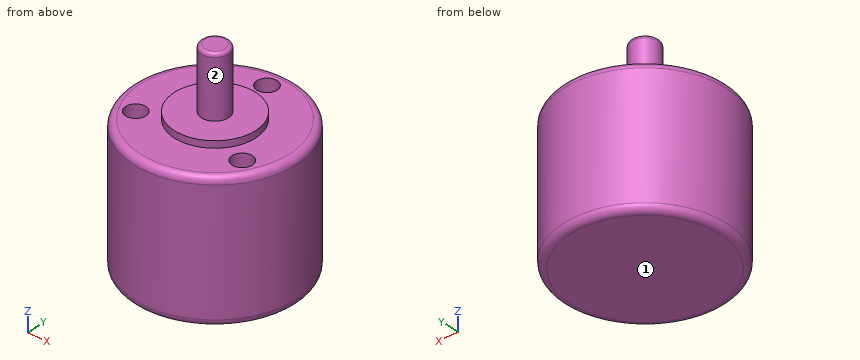
```python
from build123d import *

# Parameters (mm, degrees)
ESQUISSE1_R             = 12
EXTRUSION1_DEPTH        = 20
ESQUISSE2_R             = 2
EXTRUSION2_DEPTH        = 10
CONG_1_R                = 1
CONG_2_R                = 1
CONG_3_R                = 0.5
ESQUISSE4_R             = 6
EXTRUSION3_DEPTH        = 1
ESQUISSE5_R             = 1.5
ENL_V_MAT_EXTRU_1_DEPTH = 5


with BuildPart() as part:
    # Esquisse1 → Extrusion1 (new body)
    with BuildSketch(Plane.XY):
        Circle(ESQUISSE1_R)
    extrude(amount=-EXTRUSION1_DEPTH)

    # Esquisse2 → Extrusion2 (add)
    with BuildSketch(Plane.XY):
        Circle(ESQUISSE2_R)
    extrude(amount=EXTRUSION2_DEPTH)

    # Congé1
    cong_1_edges = [part.edges().sort_by_distance(p)[0] for p in [
        (-12, 0, 0),
    ]]
    fillet(cong_1_edges, radius=CONG_1_R)

    # Congé2
    cong_2_edges = [part.edges().sort_by_distance(p)[0] for p in [
        (-12, 0, -20),
    ]]
    fillet(cong_2_edges, radius=CONG_2_R)

    # Congé3
    cong_3_edges = [part.edges().sort_by_distance(p)[0] for p in [
        (-2, 0, 10),
    ]]
    fillet(cong_3_edges, radius=CONG_3_R)

    # Esquisse4 → Extrusion3 (add)
    with BuildSketch(Plane.XY):
        Circle(ESQUISSE4_R)
    extrude(amount=EXTRUSION3_DEPTH)

    # Esquisse5 → Enlèv. mat.-Extru.1 (cut)
    with BuildSketch(Plane.XY):
        with Locations((0, 9)):
            Circle(ESQUISSE5_R)
        with Locations((-7.794228634, -4.5)):
            Circle(ESQUISSE5_R)
        with Locations((7.794228634, -4.5)):
            Circle(ESQUISSE5_R)
    extrude(amount=-ENL_V_MAT_EXTRU_1_DEPTH, mode=Mode.SUBTRACT)


solid = part.part
```
Check sheet for the modelled part. Datum: model origin and axes. Units: mm. Face numbers are marked on the shaded views. A direction names the side the tool comes from. Round coordinates to 2 decimals unless told otherwise and drop trailing zeros. Loops run counter-clockwise (first coordinate to the right, second up) from the corner with the lowest first, then second, coordinate; pieces in that order, holes last. Notation, with made-up numbers: (-20, 56) - (23, 56) arc R13 cw to (23, 77) - close; hole circle Ø5 at (15.5, 79.5). An arc over 180 degrees is marked (long way). Answer as a JSON object with one key per item and string values. Group by question number.
Q1. Sectioned sample at C-C, the plane z = 8. Enter the section's corners in (x, y), plus the area to 3 significant figures.
Q2. Gauge pin test, flat ends, axial feed: P1, Ø8, axis at y = 9, z = -11, coming from the -X side; P2, Ø12, axis at x = -8.5, y = -0.5, coming from the +Z side; P3, Ø1, axis at x = -6.5, y = 5, coming from the +Z side. Record the tip position at first contact, or that the pin passes through.
Q3. Scan lines: line 1 along Y through (x, z) = (0, -3.2); line 2 along Y through (x, z) = (0, -18.75); line 3 along Z through (x, y) = (-3.25, -1.5). Record each from-to range of solid material in increasing order. Write a range as [from, to].
Q4. Sectioned sample at B-B, the plane y = 0. Enter the section's corners in (x, z).
Q5. Set-up check for the marked faces 1 and 2: record each of +Z, -Z, +X, -X, +Y, -Y from which the full face is reachable in a straight line by a thin tool's end or side.
Q6. Sectioned sample at A-A, the plane z = -2.75. Enter the section's corners in (x, y), plus the area to 3 significant figures.
Solution:
{
 "1": {"outline": "circle Ø4 at (0, 0)", "area": "12.6 mm²"},
 "2": {"P1": "stops at x = -10.91", "P2": "stops at z = 1", "P3": "stops at z = 0"},
 "3": {"line 1": "y = [-12, 7.5], [10.5, 12]", "line 2": "y = [-12, 12]", "line 3": "z = [-20, 1]"},
 "4": {"outline": "(-12, -19) arc R1 ccw to (-11, -20) - (11, -20) arc R1 ccw to (12, -19) - (12, -1) arc R1 ccw to (11, 0) - (6, 0) - (6, 1) - (2, 1) - (2, 9.5) arc R0.5 ccw to (1.5, 10) - (-1.5, 10) arc R0.5 ccw to (-2, 9.5) - (-2, 1) - (-6, 1) - (-6, 0) - (-11, 0) arc R1 ccw to (-12, -1) - close"},
 "5": {"face 1": "-Z, +X, -X, +Y, -Y", "face 2": "+Z"},
 "6": {"outline": "circle Ø24 at (0, 0); hole circle Ø3 at (-7.79, -4.5); hole circle Ø3 at (0, 9); hole circle Ø3 at (7.79, -4.5)", "area": "431 mm²"}
}
